```python
from build123d import *

# Parameters (mm, degrees)
MAKERBEAMFIX_DEPTH          = 12.5
SKETCH3_W                   = 25
SKETCH3_H                   = 25
SKETCH3_R                   = 10.1
MAKERBEAMTHREADINGTAP_DEPTH = 12
SKETCH4_R                   = 1.5
FIXINGHOLE_DEPTH            = 31.6
SKETCH5_R                   = 4.25
DRIVERHOLE_DEPTH            = 27.6000001


with BuildPart() as part:
    # Sketch1 → MakerBeamFix (new body, symmetric)
    with BuildSketch(Plane.XY):
        Polygon((-5, 0), (5, 0), (5, 7), (1.45, 7), (1.45, 8), (-1.45, 8), (-1.45, 7), (-5, 7), align=None)
    extrude(amount=MAKERBEAMFIX_DEPTH, both=True)

    # Sketch3 → MakerBeamThreadingTap (add)
    with BuildSketch(Plane.ZY.offset(5)):
        with Locations((0, -10.1)):
            Rectangle(SKETCH3_W, SKETCH3_H)
        with Locations((0, -10.1)):
            Circle(SKETCH3_R, mode=Mode.SUBTRACT)
    extrude(amount=-MAKERBEAMTHREADINGTAP_DEPTH)

    # Sketch4 → FixingHole (cut, through all)
    with BuildSketch(Plane.XZ.offset(22.6)):
        Circle(SKETCH4_R)
    extrude(amount=-FIXINGHOLE_DEPTH, mode=Mode.SUBTRACT)

    # Sketch5 → DriverHole (cut, through all)
    with BuildSketch(Plane(origin=(0, 4, 0), x_dir=(1, 0, 0), z_dir=(0, 1, 0))):
        Circle(SKETCH5_R)
    extrude(amount=-DRIVERHOLE_DEPTH, mode=Mode.SUBTRACT)


solid = part.part
```
Verification items for the finished model (mm, model axes). A direction names the side the tool comes from. Give positions to 0.01 mm unless a question says otherwise; leave off trailing zeros. Write each loop counter-clockwise with the first axis right and the second up, starting at its lowest first coordinate (ties: lowest second). Pieces come first, ordered by that corner, then holes. Notation, with made-up numbers: (-21, -36) - (17, -36) arc R35 ccw to (17, 0) - close; hole circle Ø6 at (8, -31). An arc over 180 degrees is marked (long way). Put each result on its own line as item: value.
Q1. Section check D-D on x = 6.25. Record the cut outline in (y, z), and give its area (3 significant figures).
Result:
outline: (-22.6, -12.5) - (2.4, -12.5) - (2.4, 12.5) - (-22.6, 12.5) - close; hole circle Ø20.2 at (-10.1, 0)
area: 305 mm2
Q2. Set-up check for faces 1 (the face through (-1.45, 7.5, 6.5)), 2 (the face through (4.054, 1.566, -1.277)), 3 (the face through (5, 5, 0)), 4 (the face through (4, -22.6, -3)): record each of +Z, -Z, +X, -X, +Y, -Y from which the full face is reachable in a straight line by a thin tool's end or side.
Result:
face 1: +Z, -Z, -X, +Y
face 2: -Y
face 3: +Z, -Z, +X, +Y
face 4: +Z, -Z, +X, -X, -Y
Q3. Depth check by flat-ended pin: P1, Ø0.8, axis at y = 7.5, z = -5, coming from the -X side; P2, Ø0.5, axis at y = 7.5, z = -5, coming from the +X side; P3, Ø2, axis at x = 5.5, z = 3.5, coming from the +Y side. Enter the tip coordinate at first touch or a pass-through.
Result:
P1: x = -1.45
P2: x = 1.45
P3: y = 7
Q4. Mould release check, pull along Y, two halves, no side actions. Record for faces 5 (the face through (0.92, -13.97, 9.33)), 6 (the face through (0, 8, -6)), 7 (the face through (1.45, 7.5, 6.5)): released by +Y, released by -Y, zero draft, split by the parting line, or undercut.
Result:
face 5: undercut
face 6: released by +Y
face 7: zero draft
Q5. Scan lines: probe 1 along Z at (x, y) = (3.75, -10.1); probe 2 along X at (y, z) = (0.6, 0); probe 3 along Z at (x, y) = (0, -21.15). Record each from-to range of solid material in increasing order. Write a range as from..to.
Result:
probe 1: -12.5..-10.1, 10.1..12.5
probe 2: -5..-4.25, 4.25..7
probe 3: -12.5..-4.25, 4.25..12.5
Q6. Section check A-A on x = 0. Record the cut outline in (y, z).
Result:
outline: (-22.6, -12.5) - (8, -12.5) - (8, -1.5) - (4, -1.5) - (4, -4.25) - (-0.94, -4.25) arc R10.1 cw to (-19.26, -4.25) - (-22.6, -4.25) - close; (-22.6, 4.25) - (-19.26, 4.25) arc R10.1 cw to (-0.94, 4.25) - (4, 4.25) - (4, 1.5) - (8, 1.5) - (8, 12.5) - (-22.6, 12.5) - close
Q7. Section check B-B on z = 0. Record the cut outline in (x, y), and give its area (3 significant figures).
Result:
outline: (-5, -22.6) - (-4.25, -22.6) - (-4.25, -20.2) - (-5, -20.2) - close; (-5, 0) - (-4.25, 0) - (-4.25, 4) - (-1.5, 4) - (-1.5, 7) - (-5, 7) - close; (1.5, 4) - (4.25, 4) - (4.25, 0) - (7, 0) - (7, 2.4) - (5, 2.4) - (5, 7) - (1.5, 7) - close; (4.25, -22.6) - (7, -22.6) - (7, -20.2) - (4.25, -20.2) - close
area: 40.2 mm2
Q8. Section check C-C on y = -10.1. Record the cut outline in (x, z).
Result:
outline: (-5, -12.5) - (7, -12.5) - (7, -10.1) - (-5, -10.1) - close; (-5, 10.1) - (7, 10.1) - (7, 12.5) - (-5, 12.5) - close
